```python
from build123d import *

# Parameters (mm, degrees)
SKIZZE1_W                       = 80
SKIZZE1_H                       = 20.2
SKIZZE1_R                       = 2.65
SKIZZE1_W_2                     = 20
SKIZZE1_H_2                     = 10
AUFSATZ_LINEAR_AUSTRAGEN1_DEPTH = 10
VERRUNDUNG1_R                   = 3
SCHNITT_LINEAR_AUSTRAGEN1_DEPTH = 1


with BuildPart() as part:
    # Skizze1 → Aufsatz-Linear austragen1 (new body)
    with BuildSketch(Plane.XY):
        with Locations((40, 10.1)):
            Rectangle(SKIZZE1_W, SKIZZE1_H)
        with Locations((15, 16.1)):
            Circle(SKIZZE1_R, mode=Mode.SUBTRACT)
        with Locations((15, 4.1)):
            Circle(SKIZZE1_R, mode=Mode.SUBTRACT)
        with Locations((65, 16.1)):
            Circle(SKIZZE1_R, mode=Mode.SUBTRACT)
        with Locations((65, 4.1)):
            Circle(SKIZZE1_R, mode=Mode.SUBTRACT)
        with Locations((40, 10.1)):
            Rectangle(SKIZZE1_W_2, SKIZZE1_H_2, mode=Mode.SUBTRACT)
    extrude(amount=AUFSATZ_LINEAR_AUSTRAGEN1_DEPTH)

    # Verrundung1
    verrundung1_edges = [part.edges().sort_by_distance(p)[0] for p in [
        (50, 5.1, 5),
        (50, 15.1, 5),
        (30, 15.1, 5),
        (30, 5.1, 5),
    ]]
    fillet(verrundung1_edges, radius=VERRUNDUNG1_R)

    # Skizze2 → Schnitt-Linear austragen1 (cut)
    with BuildSketch(Plane.XY.offset(10)):
        with BuildLine():
            Line((55.5, 12.6), (55.5, 7.6))
            ThreePointArc((55.5, 7.6), (53.449747468, 2.650252532), (48.5, 0.6))
            Line((48.5, 0.6), (31.5, 0.6))
            ThreePointArc((31.5, 0.6), (26.550252532, 2.650252532), (24.5, 7.6))
            Line((24.5, 7.6), (24.5, 12.6))
            ThreePointArc((24.5, 12.6), (26.550252532, 17.549747468), (31.5, 19.6))
            Line((31.5, 19.6), (48.5, 19.6))
            ThreePointArc((48.5, 19.6), (53.449747468, 17.549747468), (55.5, 12.6))
        make_face()
        with BuildLine():
            Line((48.5, 16.6), (31.5, 16.6))
            ThreePointArc((31.5, 16.6), (28.671572875, 15.428427125), (27.5, 12.6))
            Line((27.5, 12.6), (27.5, 7.6))
            ThreePointArc((27.5, 7.6), (28.671572875, 4.771572875), (31.5, 3.6))
            Line((31.5, 3.6), (48.5, 3.6))
            ThreePointArc((48.5, 3.6), (51.328427125, 4.771572875), (52.5, 7.6))
            Line((52.5, 7.6), (52.5, 12.6))
            ThreePointArc((52.5, 12.6), (51.328427125, 15.428427125), (48.5, 16.6))
        make_face(mode=Mode.SUBTRACT)
    extrude(amount=-SCHNITT_LINEAR_AUSTRAGEN1_DEPTH, mode=Mode.SUBTRACT)


solid = part.part
```
Geometry: final body of the model. Coordinates: model frame, mm. A direction names the side the tool comes from. Round coordinates to 2 decimals unless told otherwise and drop trailing zeros. Write each loop counter-clockwise with the first axis right and the second up, starting at its lowest first coordinate (ties: lowest second). Pieces come first, ordered by that corner, then holes. Notation, with made-up numbers: M -19.5,-10 L -10.5,-10 A21 cw -10.5,-2 Z; hole C 74,16 d10. An arc over 180 degrees is marked long. Answer in a Markdown table with one row per item. Add a question column.
(1) Cut plane A-A, the plane x = 65. Return the cut outline in (y, z), then the cut area to 3 significant figures.
(2) Cut plane D-D, the plane y = 17.5. Return the cut outline in (x, z), then the cut area to 3 significant figures.
(3) Cut plane C-C, the plane x = 45. Return the cut outline in (y, z), then the cut area to 3 significant figures.
(4) Ray query, L1, parallel to Y at x = 15, z = 2.5; L2, parallel to X at y = 11, z = 0.75; L3, parallel to X at y = 16, z = 1.75. Return the intervals inside material, ascending.
(5) Reachability of faces 4 (the face through (80, 10, 5)), 5 (the face through (49.14, 14.2, 5.07)), 6 (the face through (53.4, 17.6, 9.5)) from +Z, -Z, +X, -X, +Y, -Y: full face, straight path, thin tool, end or side. Return the list, or none.
(6) Cut plane B-B, the plane z = 5.5. Return the cut outline in (x, y).
(7) Draft query along Y for faces 1 (the face through (0, 10, 5)), 2 (the face through (51.297, 4.741, 9.507)), 3 (the face through (39, 20.2, 5)). Return one class per face: pulls with the +Y half, pulls with the -Y half, needs draft (parallel to the pull), parting line crosses it, or undercut.
Established:
| question | item | result |
|---|---|---|
| 1 | outline | M 0,0 L 1.45,0 L 1.45,10 L 0,10 Z; M 6.75,0 L 13.45,0 L 13.45,10 L 6.75,10 Z; M 18.75,0 L 20.2,0 L 20.2,10 L 18.75,10 Z |
| 1 | area | 96.0 mm² |
| 2 | outline | M 0,0 L 12.75,0 L 12.75,10 L 0,10 Z; M 17.25,0 L 62.75,0 L 62.75,10 L 53.5,10 L 53.5,9 L 26.5,9 L 26.5,10 L 17.25,10 Z; M 67.25,0 L 80,0 L 80,10 L 67.25,10 Z |
| 2 | area | 683 mm² |
| 3 | outline | M 0,0 L 5.1,0 L 5.1,10 L 3.6,10 L 3.6,9 L 0.6,9 L 0.6,10 L 0,10 Z; M 15.1,0 L 20.2,0 L 20.2,10 L 19.6,10 L 19.6,9 L 16.6,9 L 16.6,10 L 15.1,10 Z |
| 3 | area | 96.0 mm² |
| 4 | L1 | 0 to 1.45, 6.75 to 13.45, 18.75 to 20.2 |
| 4 | L2 | 0 to 30, 50 to 80 |
| 4 | L3 | 0 to 12.35, 17.65 to 62.35, 67.65 to 80 |
| 5 | face 4 | +Z, -Z, +X, +Y, -Y |
| 5 | face 5 | +Z, -Z |
| 5 | face 6 | +Z |
| 6 | outline | M 0,0 L 80,0 L 80,20.2 L 0,20.2 Z; hole C 15,4.1 d5.3; hole C 15,16.1 d5.3; hole M 30,8.1 A3 ccw 33,5.1 L 47,5.1 A3 ccw 50,8.1 L 50,12.1 A3 ccw 47,15.1 L 33,15.1 A3 ccw 30,12.1 Z; hole C 65,4.1 d5.3; hole C 65,16.1 d5.3 |
| 7 | face 1 | needs draft |
| 7 | face 2 | undercut |
| 7 | face 3 | pulls with the +Y half |
